from build123d import *

# Parameters (mm, degrees)
SKETCH1_R           = 25
SKETCH1_R_2         = 22.5
BOSS_EXTRUDE1_DEPTH = 300
SKETCH2_W           = 15
SKETCH2_H           = 7.280738242
CUT_EXTRUDE1_DEPTH  = 200
SKETCH3_R           = 25
BOSS_EXTRUDE2_DEPTH = 2.5


with BuildPart() as part:
    # Sketch1 → Boss-Extrude1 (new body)
    with BuildSketch(Plane.XY):
        Circle(SKETCH1_R)
        Circle(SKETCH1_R_2, mode=Mode.SUBTRACT)
    extrude(amount=-BOSS_EXTRUDE1_DEPTH)

    # Sketch2 → Cut-Extrude1 (cut)
    with BuildSketch(Plane.XY):
        with Locations((0, 23)):
            Rectangle(SKETCH2_W, SKETCH2_H)
    cut_extrude1 = extrude(amount=-CUT_EXTRUDE1_DEPTH, mode=Mode.SUBTRACT)

    # Mirror1: Cut-Extrude1 across plane
    add(cut_extrude1.mirror(Plane.ZX), mode=Mode.SUBTRACT)

    # Sketch3 → Boss-Extrude2 (add)
    with BuildSketch(Plane(origin=(0, 0, -300), x_dir=(-1, 0, 0), z_dir=(0, 0, -1))):
        with Locations(Location((0, 0, 0), (0, 0, 107.457603124))):
            Circle(SKETCH3_R)
    extrude(amount=BOSS_EXTRUDE2_DEPTH)


solid = part.part
Could you check a few things on this model? Use its own coordinates, in mm. A direction names the side the tool comes from. Give positions to 0.01 mm unless a question says otherwise; leave off trailing zeros. Order: outer loops, then holes, each group sorted by start corner. A loop starts at its lowest first (then second) coordinate and runs counter-clockwise, first axis right, second up.
1. Suppose I cut it at A-A (z = -76). Write out the boundary of the cut face in (x, y).
Answers below:
outline: (-7.5, -23.85) - (-7.5, -21.21) arc R22.5 cw to (-7.5, 21.21) - (-7.5, 23.85) arc R25 ccw to start; (7.5, -23.85) arc R25 ccw to (7.5, 23.85) - (7.5, 21.21) arc R22.5 cw to (7.5, -21.21) - close
2. Suppose I cut it at D-D (z = -219). Write out the boundary of the cut face in (x, y), plus the area to 3 significant figures.
Answers below:
outline: circle Ø50 at (0, 0); hole circle Ø45 at (0, 0)
area: 373 mm2
3. Suppose I cut it at C-C (y = 0). Write out the boundary of the cut face in (x, z).
Answers below:
outline: (-25, -302.5) - (25, -302.5) - (25, 0) - (22.5, 0) - (22.5, -300) - (-22.5, -300) - (-22.5, 0) - (-25, 0) - close
4. Which directions (+Z, -Z, +X, -X, +Y, -Y) give clear straight access to the entire face, cutting with the end or side of a thin tool? Please do faces 1 (the cylindrical face through (20.784, -8.618, -147.9)), 2 (the flat face through (0, 0, -302.5)).
Answers below:
face 1: +Z
face 2: -Z, +X, -X, +Y, -Y
5. Thinking about a two-plate mould opening in Y: for faces 3 (the flat face through (0, 0, -300)), 4 (the flat face through (-23, 0, 0)), which applies, +Y half, -Y half, draft (parallel to the pull), parting line (faces both ways), or undercut?
Answers below:
face 3: undercut
face 4: draft
6. Suppose I cut it at B-B (x = 0). Write out the boundary of the cut face in (y, z), plus the area to 3 significant figures.
Answers below:
outline: (-25, -302.5) - (25, -302.5) - (25, -200) - (22.5, -200) - (22.5, -300) - (-22.5, -300) - (-22.5, -200) - (-25, -200) - close
area: 625 mm2
7. I need wall thicknesses on L1, parallel to X at y = 0, z = -164; L2, parallel to Y at x = 1, z = -216; L3, parallel to Z at x = 19.5, y = 4. Which ranges of each line are inside material? Lowest first, please.
Answers below:
L1: x = -25 to -22.5, 22.5 to 25
L2: y = -24.98 to -22.48, 22.48 to 24.98
L3: z = -302.5 to -300
8. For pin 1 (1.3 mm diameter, centred on y = -23, z = -121, fed in from +X); pin 2 (2 mm diameter, centred on y = 22.5, z = -82.5, fed in from -X); pin 3 (1.1 mm diameter, centred on x = 2.5, y = -23.5, fed in from +Z), each with a flat end and sliding along its axis, tell me the tip position at first contact or that it passes through.
Answers below:
pin 1: stops at x = 11.2
pin 2: stops at x = -12.76
pin 3: stops at z = -200
